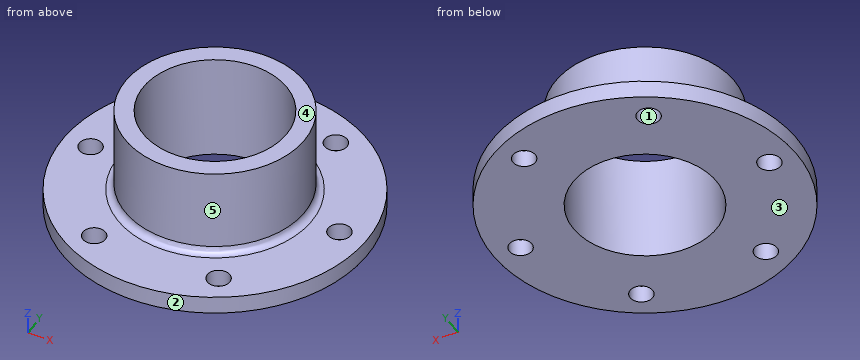
Autodesk Inventor part; units mm, degrees
ref_plane "YZ Plane" through (0, 0, 0) normal (1, 0, 0) x (0, 1, 0)
ref_plane "XZ Plane" through (0, 0, 0) normal (0, 1, 0) x (-1, 0, 0)
ref_plane "XY Plane" through (0, 0, 0) normal (0, 0, 1) x (1, 0, 0)
sketch "Sketch7" plane through (0, 0, 0) normal (0, 0, 1) x (1, 0, 0)
  circle A0 centre (0, 0) radius 42.5
  circle A1 centre (0, 0) radius 20
  dimension "d59" = 85
  dimension "d60" = 40
extrude "Extrusion6" add sketch "Sketch7" along normal blind 5
sketch "Sketch8" plane through (0, 0, 5) normal (0, 0, 1) x (1, 0, 0)
  circle A0 centre (0, 0) radius 25
  circle A1 centre (0, 0) radius 20
  dimension "d55" = 50
extrude "Extrusion7" add sketch "Sketch8" along normal blind 25
fillet "Fillet4" radius 2 1 edges at (-25, 0, 5)
sketch "Sketch9" plane through (0, 0, 5) normal (0, 0, 1) x (1, 0, 0)
  circle A0 centre (0, 0) radius 35 construction
  circle A1 centre (-35, 0) radius 3.15
  circle A2 centre (-17.5, -30.3109) radius 3.15
  circle A3 centre (17.5, -30.3109) radius 3.15
  circle A4 centre (35, 0) radius 3.15
  circle A5 centre (17.5, 30.3109) radius 3.15
  circle A6 centre (-17.5, 30.3109) radius 3.15
  dimension "d61" = 70
  dimension "d62" = 6.3
  dimension "d65" = 360
extrude "Extrusion8" cut sketch "Sketch9" against normal through all
properties part number "HOSE-NOZZLE-MOUNTING"
Could you check a few things on this model? Use its own coordinates, in mm. Face numbers are marked on the shaded views. A direction names the side the tool comes from. Coordinates: 2 decimals unless noted, no trailing zeros. Write each loop counter-clockwise with the first axis right and the second up, starting at its lowest first coordinate (ties: lowest second). Pieces come first, ordered by that corner, then holes. Notation, with made-up numbers: (23.25, -26.5) - (54.25, -26.5) arc R16 cw to (54.25, -9.5) - close; hole circle Ø8 at (16.5, 39.25). An arc over 180 degrees is marked (long way). Use a Markdown table: item, result.
Q1. Thinking about a two-plate mould opening in X: for the marked faces 1, 2 and 3, which applies, +X half, -X half, draft (parallel to the pull), parting line (faces both ways), or undercut?
Geometry check:
| item | result |
|---|---|
| face 1 | undercut |
| face 2 | parting line |
| face 3 | draft |
Q2. Imagine slicing it at B-B (x = 35). List the corners of the cut face in (y, z) for me.
Geometry check:
| item | result |
|---|---|
| outline | (-24.11, 0) - (-3.15, 0) - (-3.15, 5) - (-24.11, 5) - close; (3.15, 0) - (24.11, 0) - (24.11, 5) - (3.15, 5) - close |
Q3. Which directions (+Z, -Z, +X, -X, +Y, -Y) give clear straight access to the entire face, cutting with the end or side of a thin tool? Please do the marked faces 4 and 5.
Geometry check:
| item | result |
|---|---|
| face 4 | +Z, +X, -X, +Y, -Y |
| face 5 | +Z |
Q4. Please list where these lines run through material, in increasing order: L1, parallel to Y at x = 0, z = 10.75; L2, parallel to Y at x = 17.5, z = 2.3; L3, parallel to Z at x = -17.5, y = 35.5.
Geometry check:
| item | result |
|---|---|
| L1 | y = -25 to -20, 20 to 25 |
| L2 | y = -38.73 to -33.46, -27.16 to -9.68, 9.68 to 27.16, 33.46 to 38.73 |
| L3 | z = 0 to 5 |
Q5. I'm going to push flat-ended pins straight in: pin 1 Ø12 at (y, z) = (-15.5, 16.5) entering from +X; pin 2 Ø3 at (x, y) = (-31, 29.5) entering from +Z; pin 3 Ø8 at (x, z) = (-15.5, 16.5) entering from +Y. Where does each tip first touch, or does it pass through?
Geometry check:
| item | result |
|---|---|
| pin 1 | stops at x = 23.12 |
| pin 2 | stops at z = 5 |
| pin 3 | stops at y = 22.2 |
Q6. Imagine slicing it at C-C (z = 10). List the corners of the cut face in (x, y) for me.
Geometry check:
| item | result |
|---|---|
| outline | circle Ø50 at (0, 0); hole circle Ø40 at (0, 0) |
Q7. Imagine slicing it at D-D (x = -17.5). Count the separate pieces of the cut face and the enclosed holes in it, and give its area (3 significant figures).
Geometry check:
| item | result |
|---|---|
| separate pieces | 4 |
| enclosed holes | 0 |
| area | 638 mm2 |
Q8. Imagine slicing it at A-A (y = 0). List the corners of the cut face in (x, z) for me.
Geometry check:
| item | result |
|---|---|
| outline | (-42.5, 0) - (-38.15, 0) - (-38.15, 5) - (-42.5, 5) - close; (-31.85, 0) - (-20, 0) - (-20, 30) - (-25, 30) - (-25, 7) arc R2 cw to (-27, 5) - (-31.85, 5) - close; (20, 0) - (31.85, 0) - (31.85, 5) - (27, 5) arc R2 cw to (25, 7) - (25, 30) - (20, 30) - close; (38.15, 0) - (42.5, 0) - (42.5, 5) - (38.15, 5) - close |
